The drawing under review shows one solid part. Ordinate dimensions are in mm from its lowest x, y, z. Coordinates: 2 decimals unless noted, no trailing zeros. Write each loop counter-clockwise with the first axis right and the second up, starting at its lowest first coordinate (ties: lowest second). Pieces come first, ordered by that corner, then holes. Notation, with made-up numbers: (-21.75, -26) - (35.25, -26) arc R13 cw to (35.25, -9) - close; hole circle Ø6 at (-30, 68). An arc over 180 degrees is marked (long way). Put each result on its own line as item: value. Start each with the question number.
Item 1: Consider section B-B on z = 0.95. State how many separate pieces and enclosed holes the cut face has, then the cut area to 3 significant figures.
Item 2: Consider section A-A on y = 24. Give the boundary of the cut face in (x, z).
Item 3: Consider section C-C on x = 8.5. Give the boundary of the cut face in (y, z) (1 decimal).
Item 4: To check wall thickness, follow L1, parallel to X at y = 23, z = 1.2 (1 decimal); L2, parallel to Y at x = 18, z = 1.1 (1 decimal); L3, parallel to Y at x = 4, z = 1.1 (1 decimal). State the ranges of each line that lie inside material, in increasing order. Write a range as [from, to].
Item 5: For pin 1 (2.5 mm diameter, centred on x = 8.75, y = 8.75, fed in from -Z); pin 2 (1 mm diameter, centred on y = 25.5, z = 0.5, fed in from +X), all flat-tipped, find the tip position at first contact; note any pin that passes through.
Item 6: Consider section D-D on y = 19.5. Give the boundary of the cut face in (x, z).
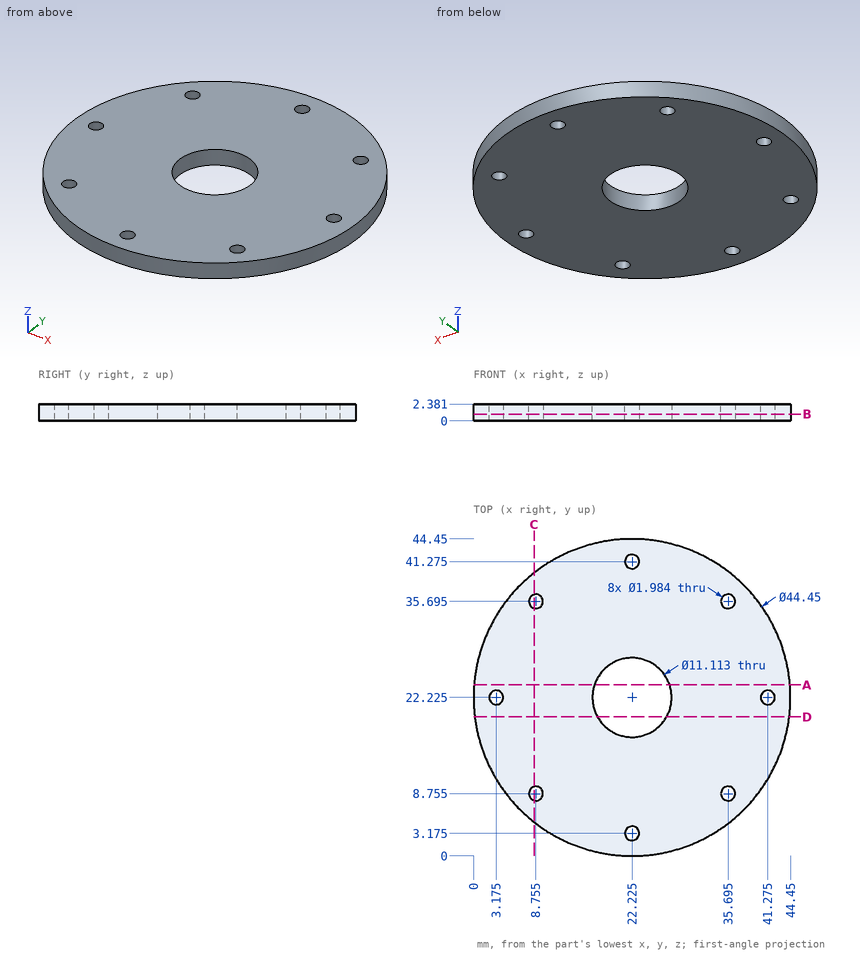
Report:
1. separate pieces: 1
1. enclosed holes: 9
1. area: 1,430 mm²
2. outline: (0.07, 0) - (16.96, 0) - (16.96, 2.38) - (0.07, 2.38) - close; (27.49, 0) - (44.38, 0) - (44.38, 2.38) - (27.49, 2.38) - close
3. outline: (4.7, 0) - (7.8, 0) - (7.8, 2.4) - (4.7, 2.4) - close; (9.7, 0) - (34.7, 0) - (34.7, 2.4) - (9.7, 2.4) - close; (36.7, 0) - (39.7, 0) - (39.7, 2.4) - (36.7, 2.4) - close
4. L1: [0, 2.6], [3.8, 16.7], [27.7, 40.7], [41.9, 44.4]
4. L2: [0.4, 18.6], [25.8, 44]
4. L3: [9.5, 21.7], [22.8, 34.9]
5. pin 1: z = 0
5. pin 2: x = 44.28
6. outline: (0.17, 0) - (17.38, 0) - (17.38, 2.38) - (0.17, 2.38) - close; (27.07, 0) - (44.28, 0) - (44.28, 2.38) - (27.07, 2.38) - close
